Part model, mm, in its own coordinate system. Face numbers are marked on the shaded views. A direction names the side the tool comes from. Round coordinates to 2 decimals unless told otherwise and drop trailing zeros. Order: outer loops, then holes, each group sorted by start corner. A loop starts at its lowest first (then second) coordinate and runs counter-clockwise, first axis right, second up. Notation, with made-up numbers: M 30.25,80 L 63.25,80 A8 ccw 63.25,91 Z; hole C 69.25,67 d6. An arc over 180 degrees is marked long. One line per question, with ' | ' between items.
from build123d import *

# Parameters (mm, degrees)
ESQUISSE1_W             = 100
ESQUISSE1_H             = 12
ESQUISSE1_R             = 2.5
BOSS_EXTRU_1_DEPTH      = 2
ESQUISSE2_W             = 100
ESQUISSE2_H             = 2
BOSS_EXTRU_2_DEPTH      = 2
ESQUISSE3_W             = 100
ESQUISSE3_H             = 4
BOSS_EXTRU_3_DEPTH      = 22
ESQUISSE4_W             = 100
ESQUISSE4_H             = 2
ENL_V_MAT_EXTRU_1_DEPTH = 6
ESQUISSE5_W             = 100
ESQUISSE5_H             = 2
BOSS_EXTRU_4_DEPTH      = 6
ESQUISSE6_W             = 100
ESQUISSE6_H             = 6
BOSS_EXTRU_5_DEPTH      = 1
ESQUISSE9_W             = 100
ESQUISSE9_H             = 1
BOSS_EXTRU_8_DEPTH      = 9
ESQUISSE10_W            = 100
ESQUISSE10_H            = 1
BOSS_EXTRU_9_DEPTH      = 1
ESQUISSE11_W            = 100
ESQUISSE11_H            = 28
ESQUISSE11_R            = 2.5
BOSS_EXTRU_10_DEPTH     = 2
ESQUISSE12_W            = 100
ESQUISSE12_H            = 28
ENL_V_MAT_EXTRU_2_DEPTH = 2
ESQUISSE13_W            = 72
ESQUISSE13_H            = 10
ENL_V_MAT_EXTRU_3_DEPTH = 2


with BuildPart() as part:
    # Esquisse1 → Boss.-Extru.1 (new body)
    with BuildSketch(Plane.XY):
        with Locations((-50, 6)):
            Rectangle(ESQUISSE1_W, ESQUISSE1_H)
        with Locations((-93, 5)):
            Circle(ESQUISSE1_R, mode=Mode.SUBTRACT)
        with Locations((-7, 5)):
            Circle(ESQUISSE1_R, mode=Mode.SUBTRACT)
    extrude(amount=BOSS_EXTRU_1_DEPTH)

    # Esquisse2 → Boss.-Extru.2 (add)
    with BuildSketch(Plane(origin=(0, 0, 0), x_dir=(-1, 0, 0), z_dir=(0, 0, -1))):
        with Locations((50, 11)):
            Rectangle(ESQUISSE2_W, ESQUISSE2_H)
    extrude(amount=BOSS_EXTRU_2_DEPTH)

    # Esquisse3 → Boss.-Extru.3 (add)
    with BuildSketch(Plane(origin=(0, 12, 0), x_dir=(1, 0, 0), z_dir=(0, 1, 0))):
        with Locations((-50, 0)):
            Rectangle(ESQUISSE3_W, ESQUISSE3_H)
    extrude(amount=BOSS_EXTRU_3_DEPTH)

    # Esquisse4 → Enlèv. mat.-Extru.1 (cut)
    with BuildSketch(Plane(origin=(0, 34, 0), x_dir=(1, 0, 0), z_dir=(0, 1, 0))):
        with Locations((-50, -1)):
            Rectangle(ESQUISSE4_W, ESQUISSE4_H)
    extrude(amount=-ENL_V_MAT_EXTRU_1_DEPTH, mode=Mode.SUBTRACT)

    # Esquisse5 → Boss.-Extru.4 (add)
    with BuildSketch(Plane(origin=(0, 0, -2), x_dir=(-1, 0, 0), z_dir=(0, 0, -1))):
        with Locations((50, 33)):
            Rectangle(ESQUISSE5_W, ESQUISSE5_H)
    extrude(amount=BOSS_EXTRU_4_DEPTH)

    # Esquisse6 → Boss.-Extru.5 (add)
    with BuildSketch(Plane(origin=(0, 0, -8), x_dir=(-1, 0, 0), z_dir=(0, 0, -1))):
        with Locations((50, 35)):
            Rectangle(ESQUISSE6_W, ESQUISSE6_H)
    extrude(amount=-BOSS_EXTRU_5_DEPTH)

    # Esquisse9 → Boss.-Extru.8 (add)
    with BuildSketch(Plane.XY.offset(-7)):
        with Locations((-50, 37.5)):
            Rectangle(ESQUISSE9_W, ESQUISSE9_H)
    extrude(amount=BOSS_EXTRU_8_DEPTH)

    # Esquisse10 → Boss.-Extru.9 (add)
    with BuildSketch(Plane.XZ.offset(-37)):
        with Locations((-50, 1.5)):
            Rectangle(ESQUISSE10_W, ESQUISSE10_H)
    extrude(amount=BOSS_EXTRU_9_DEPTH)

    # Esquisse11 → Boss.-Extru.10 (add)
    with BuildSketch(Plane(origin=(0, 0, -2), x_dir=(-1, 0, 0), z_dir=(0, 0, -1))):
        with Locations((50, 14)):
            Rectangle(ESQUISSE11_W, ESQUISSE11_H)
        with Locations((93, 5)):
            Circle(ESQUISSE11_R, mode=Mode.SUBTRACT)
        with Locations((7, 5)):
            Circle(ESQUISSE11_R, mode=Mode.SUBTRACT)
    extrude(amount=BOSS_EXTRU_10_DEPTH)

    # Esquisse12 → Enlèv. mat.-Extru.2 (cut)
    with BuildSketch(Plane.XY.offset(2)):
        with Locations((-50, 14)):
            Rectangle(ESQUISSE12_W, ESQUISSE12_H)
    extrude(amount=-ENL_V_MAT_EXTRU_2_DEPTH, mode=Mode.SUBTRACT)

    # Esquisse13 → Enlèv. mat.-Extru.3 (cut)
    with BuildSketch(Plane.XY.offset(-2)):
        with Locations((-50, 5)):
            Rectangle(ESQUISSE13_W, ESQUISSE13_H)
    extrude(amount=-ENL_V_MAT_EXTRU_3_DEPTH, mode=Mode.SUBTRACT)


solid = part.part
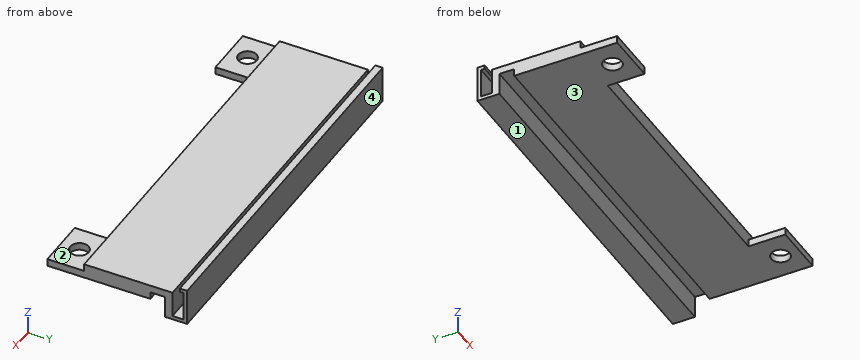
1) Drop flat-ended pins along their axis: pin 1 (1.2 mm diameter, centred on x = -55, z = -1.5, fed in from -Y); pin 2 (5 mm diameter, centred on x = -28, y = 26, fed in from -Z); pin 3 (8 mm diameter, centred on x = -3.5, y = 3, fed in from +Z); pin 4 (4 mm diameter, centred on x = -7, y = 5, fed in from -Z). Give the stop position or say it passes through.
The answers:
pin 1: stops at y = 10 | pin 2: stops at z = -4 | pin 3: stops at z = -2 | pin 4: passes through
2) Two-plate mould, pull along Y, no slides. Class the marked faces 3 and 4: released by +Y, released by -Y, zero draft, split by the parting line, or undercut.
The answers:
face 3: zero draft | face 4: released by +Y
3) Saw through at B-B (z = -5.5). List the corners of the cut face in (x, y), plus the area to 3 significant figures.
The answers:
outline: M -100,32 L 0,32 L 0,34 L -100,34 Z; M -100,37 L 0,37 L 0,38 L -100,38 Z | area: 300 mm²
4) Probe line 1 (Y direction, x = -7, z = -2.75); line 2 (Y direction, x = -22, z = -2.25); line 3 (Y direction, x = -74, z = -1.25). List the from-to ranges inside material, lowest first. Write a range as [from, to].
The answers:
line 1: y = [0, 2.5], [7.5, 28], [32, 34], [37, 38] | line 2: y = [10, 28], [32, 34], [37, 38] | line 3: y = [10, 34], [37, 38]
5) Saw through at C-C (x = -7). List the corners of the cut face in (y, z), plus the area to 3 significant figures.
The answers:
outline: M 0,-4 L 2.5,-4 L 2.5,-2 L 0,-2 Z; M 7.5,-4 L 28,-4 L 28,-2 L 32,-2 L 32,-8 L 38,-8 L 38,2 L 36,2 L 36,1 L 37,1 L 37,-7 L 34,-7 L 34,0 L 10,0 L 10,-2 L 7.5,-2 Z | area: 120 mm²
6) Saw through at D-D (x = -42). List the corners of the cut face in (y, z).
The answers:
outline: M 10,-4 L 28,-4 L 28,-2 L 32,-2 L 32,-8 L 38,-8 L 38,2 L 36,2 L 36,1 L 37,1 L 37,-7 L 34,-7 L 34,0 L 10,0 Z
7) Saw through at A-A (y = 5). List the corners of the cut face in (x, z), plus the area to 3 significant figures.
The answers:
outline: M -100,-4 L -95.5,-4 L -95.5,-2 L -100,-2 Z; M -90.5,-4 L -86,-4 L -86,-2 L -90.5,-2 Z; M -14,-4 L -9.5,-4 L -9.5,-2 L -14,-2 Z; M -4.5,-4 L 0,-4 L 0,-2 L -4.5,-2 Z | area: 36.0 mm²
8) Which spindle directions (+Z, -Z, +X, -X, +Y, -Y) get a long thin tool onto all of the face, cutting with end or side? Do the marked faces 1 and 2. Say none if no direction does.
The answers:
face 1: -Z, +X, -X, +Y, -Y | face 2: +Z, +X, -X, -Y
